Here's how the part is built. I have some questions about the finished solid (model axes, mm). Round coordinates to 2 decimals unless told otherwise and drop trailing zeros. Order: outer loops, then holes, each group sorted by start corner. A loop starts at its lowest first (then second) coordinate and runs counter-clockwise, first axis right, second up. Notation, with made-up numbers: M 61,-35.5 L 84,-35.5 A27 ccw 84,-19.5 Z; hole C -21,89 d10. An arc over 180 degrees is marked long. Write item = value, one per line. Start each with the question number.
Item 1: I want a section at C-C, the plane x = -44. List the corners of the cut face in (y, z) for me.
Item 2: I want a section at B-B, the plane x = -33.5. List the corners of the cut face in (y, z) for me.
Item 3: I'm going to push a flat-ended pin straight in: P1, Ø6, axis at x = -35, y = -20.5, coming from the -Z side. Where does the tip first touch, or does it pass through?
Item 4: Please list where these lines run through material, in increasing order: L1, parallel to X at y = -13.25, z = 2.7; L2, parallel to X at y = -10, z = 0.6; L3, parallel to Y at x = -7, z = 0.1.
```python
from build123d import *

# Parameters (mm, degrees)
EXTRU_MINCE1_DEPTH      = 3
CONG_1_R                = 5
ESQUISSE2_R             = 7.5
BOSS_EXTRU_1_DEPTH      = 3
ESQUISSE3_R             = 4.35
ENL_V_MAT_EXTRU_1_DEPTH = 6
ENL_V_MAT_EXTRU_2_DEPTH = 10


with BuildPart() as part:
    # Esquisse1 → Extru.-Mince1 (new body)
    with BuildSketch(Plane.XY):
        with BuildLine():
            Line((-70, 0), (-48.719716507, -16.290501455))
            ThreePointArc((-48.719716507, -16.290501455), (-37.196582195, -20.399539826), (-25.436213508, -17.028998471))
            Line((-25.436213508, -17.028998471), (0, 0))
            Line((0, 0), (5.563167687, -8.309703081))
            Line((5.563167687, -8.309703081), (-19.873045821, -25.338701551))
            ThreePointArc((-19.873045821, -25.338701551), (-37.513598853, -30.394513585), (-54.79830032, -24.230956028))
            Line((-54.79830032, -24.230956028), (-76.078583813, -7.940454573))
            Line((-76.078583813, -7.940454573), (-70, 0))
        make_face()
    extrude(amount=EXTRU_MINCE1_DEPTH)

    # Congé1
    cong_1_edges = [part.edges().sort_by_distance(p)[0] for p in [
        (-76.078583813, -7.940454573, 1.5),
        (5.563167687, -8.309703081, 1.5),
        (0, 0, 1.5),
    ]]
    fillet(cong_1_edges, radius=CONG_1_R - 0.0001)  # a hair under: the kernel refuses the full size

    # Esquisse2 → Boss.-Extru.1 (add)
    with BuildSketch(Plane.XY.offset(3)):
        with Locations((-5.528119238, -9.718019227)):
            Circle(ESQUISSE2_R)
    extrude(amount=-BOSS_EXTRU_1_DEPTH)

    # Esquisse3 → Enlèv. mat.-Extru.1 (cut)
    with BuildSketch(Plane.XY.offset(3)):
        with Locations((-5.528119238, -9.718019227)):
            Circle(ESQUISSE3_R)
    extrude(amount=-ENL_V_MAT_EXTRU_1_DEPTH, mode=Mode.SUBTRACT)

    # Esquisse4 → Enlèv. mat.-Extru.2 (cut)
    with BuildSketch(Plane.XY.offset(3)):
        Polygon((-73.230010145, -4.219362538), (-65.186412562, -3.684901716), (-70, 0), align=None)
    extrude(amount=-ENL_V_MAT_EXTRU_2_DEPTH, mode=Mode.SUBTRACT)


solid = part.part
```
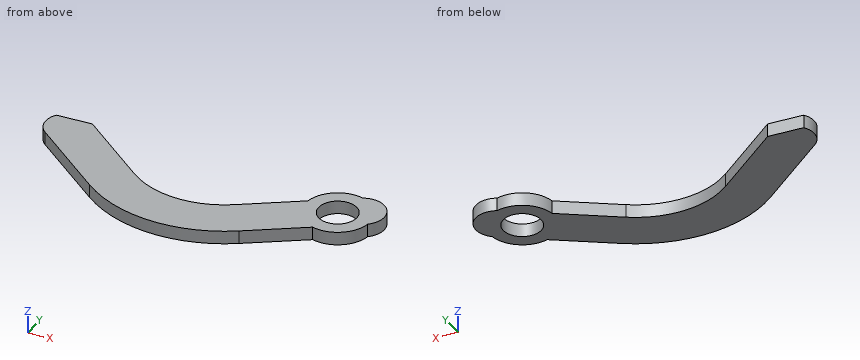
Filled in:
q1.outline = M -29.47,0 L -18.98,0 L -18.98,3 L -29.47,3 Z
q2.outline = M -30.25,0 L -20.17,0 L -20.17,3 L -30.25,3 Z
q3.P1 = 0
q4.L1 = -69.14 to -52.69, -19.79 to -8.07, -2.99 to 1.09
q4.L2 = -73.08 to -56.94, -14.94 to -9.87, -1.19 to 2.58
q4.L3 = -17.07 to -13.81, -5.62 to -2.36
